Input: part model. Units: mm. Frame: model coordinates. Face numbers are marked on the shaded views. A direction names the side the tool comes from. Coordinates: 2 decimals unless noted, no trailing zeros. Write each loop counter-clockwise with the first axis right and the second up, starting at its lowest first coordinate (ties: lowest second). Pieces come first, ordered by that corner, then holes.
1) Section query A-A (y = -2.5). Output: boundary loops of the cut face in (x, z).
2) Section query B-B (z = 0). Output: boundary loops of the cut face in (x, y) (3 decimals).
3) Section query C-C (y = -18.5). Output: boundary loops of the cut face in (x, z).
4) Line query: L1, parallel to Y at x = 0, z = 6.5; L2, parallel to Y at x = 5.25, z = 2; L3, parallel to Z at x = 0.25, y = -8.5. Output: solid intervals per line, ascending.
5) Pin query (flat end, axial travel): pin 1 Ø1 at (y, z) = (-18.5, -1.5) entering from -X; pin 2 Ø6 at (y, z) = (-15, 3) entering from -X; pin 3 Ø4 at (x, y) = (-2.5, -12) entering from +Z. Return the tip coordinate at first contact, or that it passes through.
6) Set-up query: the marked faces 1 and 2. Return all of +Z, -Z, +X, -X, +Y, -Y with unobstructed straight access to the full face (end or side cutting, diameter ignored); none if empty.
Autodesk Inventor part; units mm, degrees
ref_plane "YZ Plane" through (0, 0, 0) normal (1, 0, 0) x (0, 1, 0)
ref_plane "XZ Plane" through (0, 0, 0) normal (0, 1, 0) x (-1, 0, 0)
ref_plane "XY Plane" through (0, 0, 0) normal (0, 0, 1) x (1, 0, 0)
sketch "Sketch1" plane through (0, 0, 0) normal (0, 0, 1) x (1, 0, 0)
  line L0 (0, 0) -> (6.175, 0)
  line L1 (9.75, -2.064) -> (9.75, -4.7)
  line L2 (5.75, -5.3) -> (4, -5.3)
  line L3 (4, -5.3) -> (4, -21.3)
  line L4 (4, -21.3) -> (0, -21.3)
  line L5 (0, -21.3) -> (0, 0)
  line L6 (5.75, -5.3) -> (5.75, -4.7)
  line L7 (5.75, -4.7) -> (9.75, -4.7)
  line L8 (6.175, 0) -> (9.75, -2.064)
  dimension "d0" = 19.5
  dimension "d1" = 8
  dimension "d3" = 16
  dimension "d4" = 11.5
  dimension "d5" = 0.6
  dimension "d22" = 30
  dimension "d23" = 12.35
  dimension "d24" = 5.3
revolve "Revolution1" add sketch "Sketch1" angle 360 about axis through (0, -21.3, 0) along (0, 1, 0)
sketch "Sketch2" plane through (0, 0, 0) normal (0, 1, 0) x (1, 0, 0)
  line L0 (0, -7.5056) -> (-6.5, -3.7528)
  line L1 (-6.5, -3.7528) -> (-6.5, 3.7528)
  line L2 (-6.5, 3.7528) -> (0, 7.5056)
  line L3 (0, 7.5056) -> (6.5, 3.7528)
  line L4 (6.5, 3.7528) -> (6.5, -3.7528)
  line L5 (6.5, -3.7528) -> (0, -7.5056)
  circle A0 centre (0, 0) radius 9.75
  point P0 (0, 0)
  point P1 (0, 0)
  dimension "d25" = 13
extrude "Extrusion1" cut sketch "Sketch2" against normal blind 5.3
thread "Thread1"
chamfer "Chamfer1" distance 0.6667 angle 45 1 edges at (-4, -21.3, 0)
equation "\"d0\" = 1.5 * S_"
equation "\"d1\" = d1_"
equation "\"d3\" = L"
equation "\"d4\" = dw"
equation "\"d5\" = hw"
equation "\"d23\" = 0.95 * S_"
equation "\"d24\" = k"
equation "\"d14\" = b"
equation "\"d16\" = 0.0833333 * d"
equation "\"d25\" = S_"
equation "\"d26\" = k"
equation "\"d\" = 8"
equation "\"d1_\" = 8"
equation "\"S_\" = 13"
equation "\"k\" = 5.3"
equation "\"e\" = 14.2"
equation "\"L\" = 16"
equation "\"b\" = 15"
equation "\"Grip_Length\" = 1"
equation "\"dw\" = 11.5"
equation "\"hw\" = 0.6"
properties part number "Bolt A M8-6g×16(S13) GOST 7798-70" material "Steel, Mild"
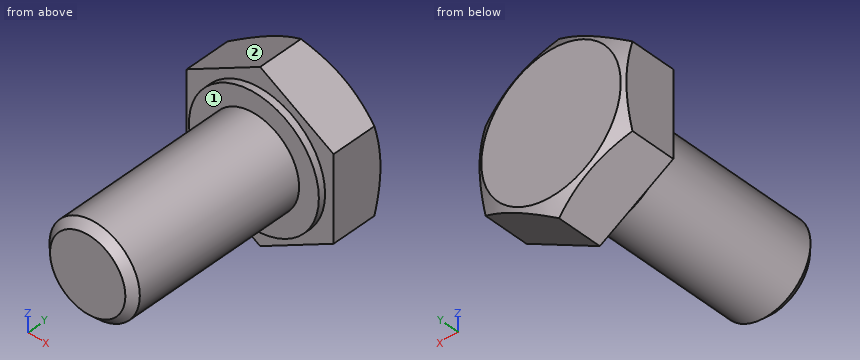
Answer:
1. outline: (-6.5, -3.75) - (0, -7.51) - (6.5, -3.75) - (6.5, 3.75) - (0, 7.51) - (-6.5, 3.75) - close
2. outline: (-6.5, -4.7) - (-5.75, -4.7) - (-5.75, -5.3) - (-4, -5.3) - (-4, -20.633) - (-3.333, -21.3) - (3.333, -21.3) - (4, -20.633) - (4, -5.3) - (5.75, -5.3) - (5.75, -4.7) - (6.5, -4.7) - (6.5, -0.188) - (6.175, 0) - (-6.175, 0) - (-6.5, -0.188) - close
3. outline: circle Ø8 at (0, 0)
4. L1: y = -4.7 to -0.19
4. L2: y = -5.3 to 0
4. L3: z = -3.99 to 3.99
5. pin 1: stops at x = -3.87
5. pin 2: stops at x = -4
5. pin 3: stops at z = 3.97
6. face 1: -Y
6. face 2: +Z, -X, +Y, -Y
